Here's the drawing with two shaded views (mm, measured from the low corner). I have some questions. Coordinates: 2 decimals unless noted, no trailing zeros. Write each loop counter-clockwise with the first axis right and the second up, starting at its lowest first coordinate (ties: lowest second). Pieces come first, ordered by that corner, then holes. Notation, with made-up numbers: (-25.75, 26.5) -> (2.25, 26.5) arc R3 ccw to (2.25, 31.5) -> close; hole circle Ø3 at (-36.75, 89). An arc over 180 degrees is marked (long way). Put each result on its own line as item: value. Start each with the question number.
Item 1: I want a section at D-D, the plane x = 57.5. List the corners of the cut face in (y, z) for me, then the cut area to 3 significant figures.
Item 2: I want a section at A-A, the plane x = 180. List the corners of the cut face in (y, z) for me, then the cut area to 3 significant figures.
Item 3: For pin 1 (2 mm diameter, centred on x = 153.5, z = 9.5, fed in from -Y) (1 decimal); pin 2 (6 mm diameter, centred on x = 196.5, z = 10, fed in from +Y) (1 decimal); pin 3 (7.5 mm diameter, centred on x = 180.5, y = 15.5, fed in from +Z), each with a flat end and sliding along its axis, tell me the tip position at first contact or that it passes through.
Item 4: I want a section at C-C, the plane z = 7.5. List the corners of the cut face in (x, y) for me, then the cut area to 3 significant figures.
Item 5: I need wall thicknesses on line 1 (Y direction, x = 180, z = 2.75); line 2 (X direction, y = 17, z = 11.4); line 3 (X direction, y = 46.5, z = 11.5). Which ranges of each line are inside material? Lowest first, please. Write a range as [from, to].
Item 6: I want a section at B-B, the plane y = 50. List the corners of the cut face in (x, z) for me, then the cut area to 3 significant figures.
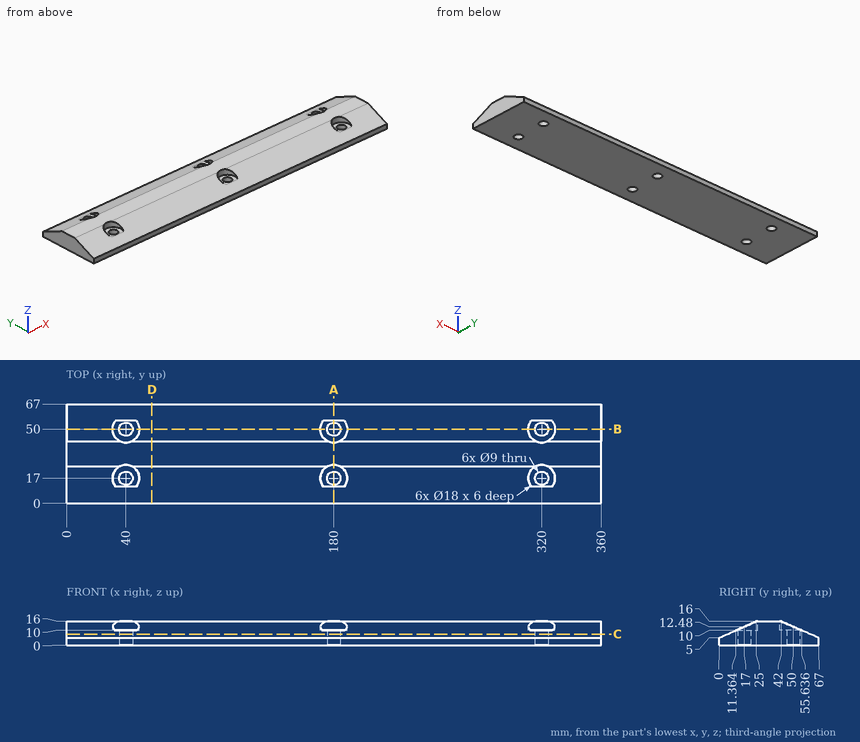
Calculated:
1. outline: (0, 0) -> (67, 0) -> (67, 5) -> (42, 16) -> (25, 16) -> (0, 5) -> close
1. area: 797 mm2
2. outline: (0, 0) -> (12.5, 0) -> (12.5, 10) -> (11.36, 10) -> (0, 5) -> close; (21.5, 0) -> (45.5, 0) -> (45.5, 10) -> (41, 10) -> (41, 16) -> (26, 16) -> (26, 10) -> (21.5, 10) -> close; (54.5, 0) -> (67, 0) -> (67, 5) -> (55.64, 10) -> (54.5, 10) -> close
2. area: 523 mm2
3. pin 1: stops at y = 8
3. pin 2: stops at y = 62.5
3. pin 3: stops at z = 10
4. outline: (0, 5.68) -> (360, 5.68) -> (360, 61.32) -> (0, 61.32) -> close; hole circle Ø9 at (40, 17); hole circle Ø9 at (40, 50); hole circle Ø9 at (180, 17); hole circle Ø9 at (180, 50); hole circle Ø9 at (320, 17); hole circle Ø9 at (320, 50)
4. area: 19,600 mm2
5. line 1: y = [0, 12.5], [21.5, 45.5], [54.5, 67]
5. line 2: x = [0, 31], [49, 171], [189, 311], [329, 360]
5. line 3: x = [0, 31.71], [48.29, 171.71], [188.29, 311.71], [328.29, 360]
6. outline: (0, 0) -> (35.5, 0) -> (35.5, 10) -> (31, 10) -> (31, 12.48) -> (0, 12.48) -> close; (44.5, 0) -> (175.5, 0) -> (175.5, 10) -> (171, 10) -> (171, 12.48) -> (49, 12.48) -> (49, 10) -> (44.5, 10) -> close; (184.5, 0) -> (315.5, 0) -> (315.5, 10) -> (311, 10) -> (311, 12.48) -> (189, 12.48) -> (189, 10) -> (184.5, 10) -> close; (324.5, 0) -> (360, 0) -> (360, 12.48) -> (329, 12.48) -> (329, 10) -> (324.5, 10) -> close
6. area: 4,090 mm2
